Geometry check sheet. Reference: the model listing, model coordinates, mm. A direction names the side the tool comes from. Coordinates: 2 decimals unless noted, no trailing zeros. Loops run counter-clockwise (first coordinate to the right, second up) from the corner with the lowest first, then second, coordinate; pieces in that order, holes last. Notation, with made-up numbers: M 81,62 L 103,62 A15 ccw 103,80 Z; hole C 87,-29.5 d2. An arc over 180 degrees is marked long. Use CSV: the item, a comma, the result in double quotes.
```python
from build123d import *

# Parameters (mm, degrees)
SKETCH1_W           = 15.106784102
SKETCH1_H           = 35.249746584
BOSS_EXTRUDE1_DEPTH = 2
SKETCH2_R           = 1.880080874
SKETCH2_R_2         = 2.135178256
BOSS_EXTRUDE2_DEPTH = 3
FILLET1_R           = 1.5


with BuildPart() as part:
    # Sketch1 → Boss-Extrude1 (new body)
    with BuildSketch(Plane.XY):
        Rectangle(SKETCH1_W, SKETCH1_H)
    extrude(amount=BOSS_EXTRUDE1_DEPTH)

    # Sketch2 → Boss-Extrude2 (add)
    with BuildSketch(Plane(origin=(0, 0, 0), x_dir=(-1, 0, 0), z_dir=(0, 0, -1))):
        with Locations((0, 10.541590628)):
            Circle(SKETCH2_R)
        Circle(SKETCH2_R_2)
    extrude(amount=BOSS_EXTRUDE2_DEPTH)

    # Fillet1
    fillet1_edges = [part.edges().sort_by_distance(p)[0] for p in [
        (1.880080874, 10.541590628, -3),
        (2.135178256, 0, -3),
    ]]
    fillet(fillet1_edges, radius=FILLET1_R)


solid = part.part
```
1. Thickness scan on line 1 (Z direction, x = -5, y = -15); line 2 (Y direction, x = 0.5, z = -2.25); line 3 (Y direction, x = -1, z = -2.35). Record the ranges inside material, lowest first. Write a range as [from, to].
The answers:
line 1,"[0, 2]"
line 2,"[-1.87, 1.87], [8.94, 12.14]"
line 3,"[-1.58, 1.58], [9.27, 11.81]"
2. Set-up check for faces 1 (the cylindrical face through (0.278, 2.117, -0.74)), 2 (the flat face through (0, 0, -3)): record each of +Z, -Z, +X, -X, +Y, -Y from which the full face is reachable in a straight line by a thin tool's end or side.
The answers:
face 1,"-Z"
face 2,"-Z, +X, -X, +Y, -Y"
3. Release check for a two-part mould opening along Y. For faces 3 (the flat face through (-7.553, 0, 1)), 4 (the cylindrical face through (0.245, 12.406, -0.74)), 5 (the flat face through (0, -17.625, 1)) record: +Y half, -Y half, draft (parallel to the pull), parting line (faces both ways), or undercut.
The answers:
face 3,"draft"
face 4,"undercut"
face 5,"-Y half"
4. Section check A-A, the plane y = -5.5. Record the cut outline in (x, z).
The answers:
outline,"M -7.55,0 L 7.55,0 L 7.55,2 L -7.55,2 Z"
5. Section check B-B, the plane x = 5.75. Record the cut outline in (y, z).
The answers:
outline,"M -17.62,0 L 17.62,0 L 17.62,2 L -17.62,2 Z"
6. Gauge pin test, flat ends, axial feed: P1, Ø2, axis at y = 8, z = -1.5, coming from the -X side; P2, Ø2, axis at x = -0.5, z = -1.5, coming from the -Y side. Record the tip position at first contact, or that the pin passes through.
The answers:
P1,"x = -1.08"
P2,"y = -2.14"
